from build123d import *

# Parameters (mm, degrees)
BOSS_EXTRUDE1_DEPTH = 20


with BuildPart() as part:
    # Sketch1 → Boss-Extrude1 (new body)
    with BuildSketch(Plane(origin=(0, 0, 0), x_dir=(1, 0, 0), z_dir=(0, 1, 0))):
        with BuildLine():
            Line((0, 214), (0, 50))
            ThreePointArc((0, 50), (-35.355339059, -35.355339059), (50, 0))
            Line((50, 0), (214, 0))
            Line((214, 0), (214, 164))
            ThreePointArc((214, 164), (249.355339059, 249.355339059), (164, 214))
            Line((164, 214), (0, 214))
        make_face()
        with BuildLine():
            Line((15, 199), (15, 31.622776602))
            ThreePointArc((15, 31.622776602), (-24.748737342, -24.748737342), (31.622776602, 15))
            Line((31.622776602, 15), (199, 15))
            Line((199, 15), (199, 182.377223398))
            ThreePointArc((199, 182.377223398), (238.748737342, 238.748737342), (182.377223398, 199))
            Line((182.377223398, 199), (15, 199))
        make_face(mode=Mode.SUBTRACT)
    extrude(amount=BOSS_EXTRUDE1_DEPTH)


solid = part.part
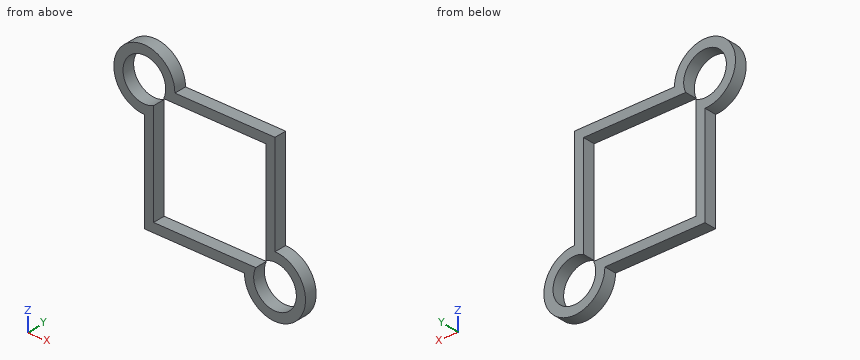
Source: CAD feature listing. Evaluate the final solid. Frame: model axes, mm. Round coordinates to 2 decimals unless told otherwise and drop trailing zeros. Loops run counter-clockwise (first coordinate to the right, second up) from the corner with the lowest first, then second, coordinate; pieces in that order, holes last. Notation, with made-up numbers: (87.25, 9.25) -> (125.25, 9.25) arc R24 ccw to (125.25, 34.25) -> close; hole circle Ø7 at (64, 86.25). An arc over 180 degrees is marked (long way). Answer as a JSON object with one key per item and string values. Group by question number.
Q1. Contact query for flat-ended pins moving along their axis: P1, Ø10, axis at y = 7.5, z = -113.5, coming from the -X side; P2, Ø5, axis at x = 103.5, y = 6, coming from the +Z side; P3, Ø6, axis at x = 74.5, y = 7, coming from the -Z side. Output: stop coordinate, or through.
Q2. Section query A-A (x = 158). Output: boundary loops of the cut face in (y, z).
Q3. Section query C-C (y = 4.25). Output: boundary loops of the cut face in (x, z).
Q4. Ray query, line 1 (Z direction, x = 154.5, y = 11); line 2 (X direction, y = 13, z = -114); line 3 (Z direction, x = 5, y = 15.75). Return the intervals inside material, ascending. Write a range as from..to.
Q5. Section query B-B (z = -126.5). Output: boundary loops of the cut face in (x, y), plus the area to 3 significant figures.
Completed:
{
 "1": {"P1": "x = 0", "P2": "z = 0", "P3": "z = -214"},
 "2": {"outline": "(0, -214) -> (20, -214) -> (20, -199) -> (0, -199) -> close; (0, -15) -> (20, -15) -> (20, 0) -> (0, 0) -> close"},
 "3": {"outline": "(0, -214) -> (164, -214) arc R50 ccw (long way) to (214, -164) -> (214, 0) -> (50, 0) arc R50 ccw (long way) to (0, -50) -> close; hole (15, -199) -> (182.38, -199) arc R35 ccw (long way) to (199, -182.38) -> (199, -15) -> (31.62, -15) arc R35 ccw (long way) to (15, -31.62) -> close"},
 "4": {"line 1": "-214..-199, -15..0", "line 2": "0..15, 199..214", "line 3": "-214..-34.64, 34.64..49.75"},
 "5": {"outline": "(0, 0) -> (15, 0) -> (15, 20) -> (0, 20) -> close; (199, 0) -> (214, 0) -> (214, 20) -> (199, 20) -> close", "area": "600 mm²"}
}
